Input: dimensioned drawing with shaded views. Units: mm. Origin: part minimum x, y, z. A direction names the side the tool comes from. Round coordinates to 2 decimals unless told otherwise and drop trailing zeros. Loops run counter-clockwise (first coordinate to the right, second up) from the corner with the lowest first, then second, coordinate; pieces in that order, holes last. Notation, with made-up numbers: M 44.25,41 L 88.25,41 A27 ccw 88.25,80 Z; hole C 42.25,3 d6. An arc over 180 degrees is marked long. Answer as CSV lines item,"result". Start each with the question number.
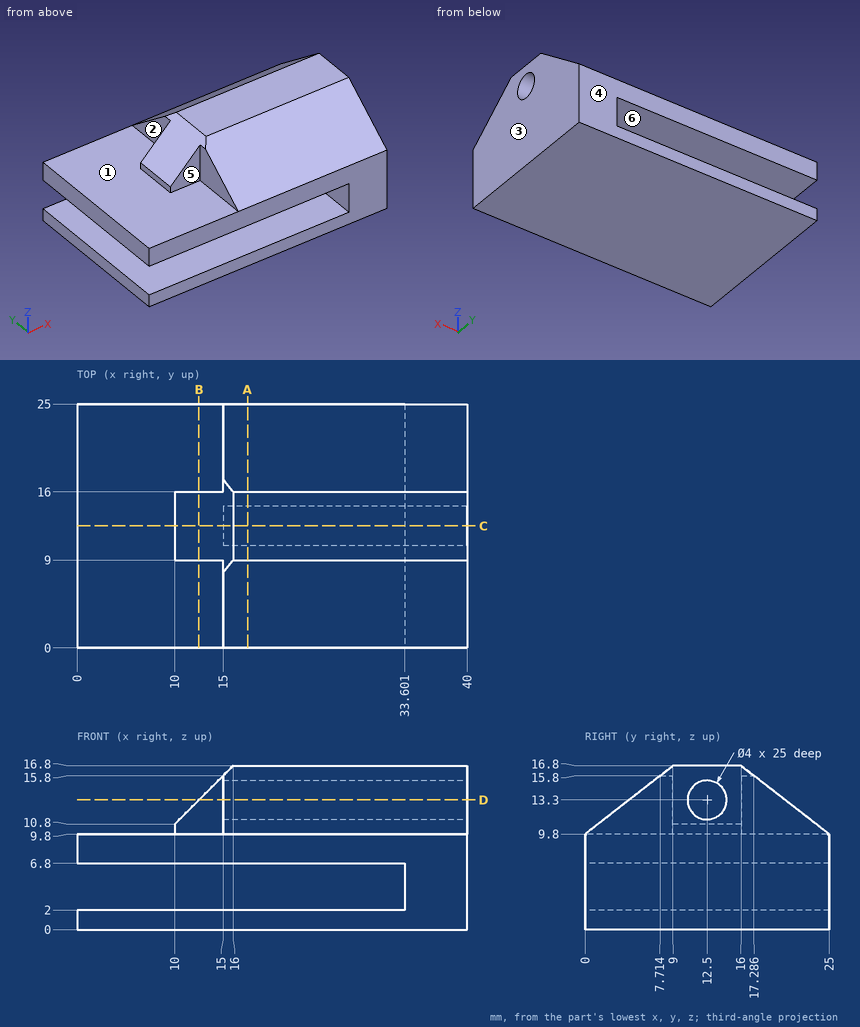
1) Section B-B, the plane x = 12.5. Return loops of the section in (y, z).
2) Section C-C, the plane y = 12.5. Return loops of the section in (x, z), and give its area (3 significant figures).
3) Section D-D, the plane z = 13.3. Return loops of the section in (x, y).
4) Mould query, pull axis X, two halves, no side actions, for the marked faces 1, 2 and 3. Classes: pulls with the +X half, pulls with the -X half, needs draft (parallel to the pull), parting line crosses it, or undercut.
5) Contact query for flat-ended pins moving along their axis: pin 1 Ø4.5 at (y, z) = (12.5, 13.3) entering from -X; pin 2 Ø12 at (x, y) = (7.5, 9.5) entering from +Z; pin 3 Ø3 at (x, z) = (29, 14.5) entering from +Y (1 decimal). Output: stop coordinate, or through.
6) Access query for the marked faces 4, 5 and 6. Directions: +Z, -Z, +X, -X, +Y, -Y. A direction counts if a zero-diameter tool reaches every point of the face in a straight line with its end or side. Return the directions, or none.
7) Section A-A, the plane x = 17.5. Return loops of the section in (y, z).
8) Ray query, line 1 along Z through (x, y) = (25.75, 12.5); line 2 along Z through (x, y) = (3, 23.25); line 3 along X through (y, z) = (5.5, 10). Return the intervals inside material, ascending.
Findings below:
1,outline,"M 0,0 L 25,0 L 25,2 L 0,2 Z; M 0,6.8 L 25,6.8 L 25,9.8 L 16,9.8 L 16,13.3 L 9,13.3 L 9,9.8 L 0,9.8 Z"
2,outline,"M 0,0 L 40,0 L 40,11.3 L 15,11.3 L 15,15.3 L 40,15.3 L 40,16.8 L 16,16.8 L 10,10.8 L 10,9.8 L 0,9.8 L 0,6.8 L 33.6,6.8 L 33.6,2 L 0,2 Z"
2,area,"323 mm²"
3,outline,"M 12.5,9 L 15,9 L 15,4.5 L 40,4.5 L 40,10.5 L 15,10.5 L 15,14.5 L 40,14.5 L 40,20.5 L 15,20.5 L 15,16 L 12.5,16 Z"
4,face 1,"needs draft"
4,face 2,"pulls with the -X half"
4,face 3,"pulls with the +X half"
5,pin 1,"x = 10.25"
5,pin 2,"z = 14.3"
5,pin 3,"y = 20.9"
6,face 4,"+Z, -Z, +X, -X, +Y"
6,face 5,"+Z, -X, -Y"
6,face 6,"-X, +Y, -Y"
7,outline,"M 0,0 L 25,0 L 25,2 L 0,2 Z; M 0,6.8 L 25,6.8 L 25,9.8 L 16,16.8 L 9,16.8 L 0,9.8 Z; hole C 12.5,13.3 d4"
8,line 1,"0 to 2, 6.8 to 11.3, 15.3 to 16.8"
8,line 2,"0 to 2, 6.8 to 9.8"
8,line 3,"15 to 40"
